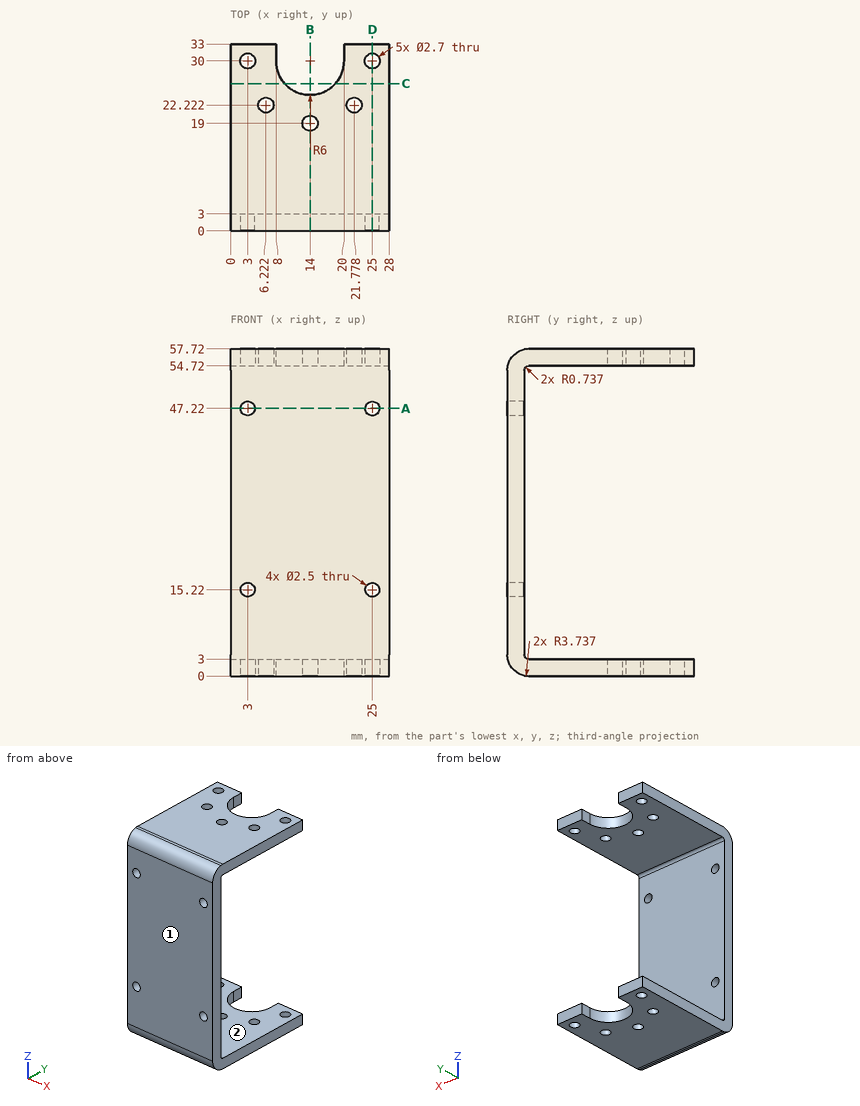
Study the drawing (mm; zero at the part's minimum x, y, z) and answer. A direction names the side the tool comes from. Round coordinates to 2 decimals unless told otherwise and drop trailing zeros. Write each loop counter-clockwise with the first axis right and the second up, starting at its lowest first coordinate (ties: lowest second). Pieces come first, ordered by that corner, then holes.
1) A cutting plane is placed at D-D (x = 25). Give the vertices of the cut face in (y, z).
2) A cutting plane is placed at A-A (z = 47.22). Give the vertices of the cut face in (x, y).
3) A cutting plane is placed at C-C (y = 26). Give the vertices of the cut face in (x, z).
4) A cutting plane is placed at B-B (x = 14). Give the vertices of the cut face in (y, z).
5) Given pin 1 Ø3 at (x, z) = (3, 46.5) entering from +Y, flat-ended and moving along its own axis, determine where the tip first touches the part or whether it passes through.
6) Straight lines are drawn through the part: line 1 (X direction, y = 30, z = 1); line 2 (Z direction, x = 5.75, y = 27); line 3 (Y direction, x = 11.75, z = 48). For each, find the intervals that lie inside material, in ascending order.
7) A tool of negligible diameter and unlimited length cuts with its end or side. For the marked faces 1 and 2, from which of +Z, -Z, +X, -X, +Y, -Y can it reach the whole face along a straight path? Write none if from no direction.
Completed:
1. outline: (0, 3.74) arc R3.74 ccw to (3.74, 0) - (28.65, 0) - (28.65, 3) - (3.74, 3) arc R0.74 cw to (3, 3.74) - (3, 13.97) - (0, 13.97) - close; (0, 16.47) - (3, 16.47) - (3, 45.97) - (0, 45.97) - close; (0, 48.47) - (3, 48.47) - (3, 53.98) arc R0.74 cw to (3.74, 54.72) - (28.65, 54.72) - (28.65, 57.72) - (3.74, 57.72) arc R3.74 ccw to (0, 53.98) - close; (31.35, 0) - (33, 0) - (33, 3) - (31.35, 3) - close; (31.35, 54.72) - (33, 54.72) - (33, 57.72) - (31.35, 57.72) - close
2. outline: (0, 0) - (1.75, 0) - (1.75, 3) - (0, 3) - close; (4.25, 0) - (23.75, 0) - (23.75, 3) - (4.25, 3) - close; (26.25, 0) - (28, 0) - (28, 3) - (26.25, 3) - close
3. outline: (0, 0) - (9.53, 0) - (9.53, 3) - (0, 3) - close; (0, 54.72) - (9.53, 54.72) - (9.53, 57.72) - (0, 57.72) - close; (18.47, 0) - (28, 0) - (28, 3) - (18.47, 3) - close; (18.47, 54.72) - (28, 54.72) - (28, 57.72) - (18.47, 57.72) - close
4. outline: (0, 3.74) arc R3.74 ccw to (3.74, 0) - (17.65, 0) - (17.65, 3) - (3.74, 3) arc R0.74 cw to (3, 3.74) - (3, 53.98) arc R0.74 cw to (3.74, 54.72) - (17.65, 54.72) - (17.65, 57.72) - (3.74, 57.72) arc R3.74 ccw to (0, 53.98) - close; (20.35, 0) - (24, 0) - (24, 3) - (20.35, 3) - close; (20.35, 54.72) - (24, 54.72) - (24, 57.72) - (20.35, 57.72) - close
5. pin 1: stops at y = 3
6. line 1: x = 0 to 1.65, 4.35 to 8, 20 to 23.65, 26.35 to 28
6. line 2: z = 0 to 3, 54.72 to 57.72
6. line 3: y = 0 to 3
7. face 1: +Z, -Z, +X, -X, -Y
7. face 2: +X, -X, +Y
